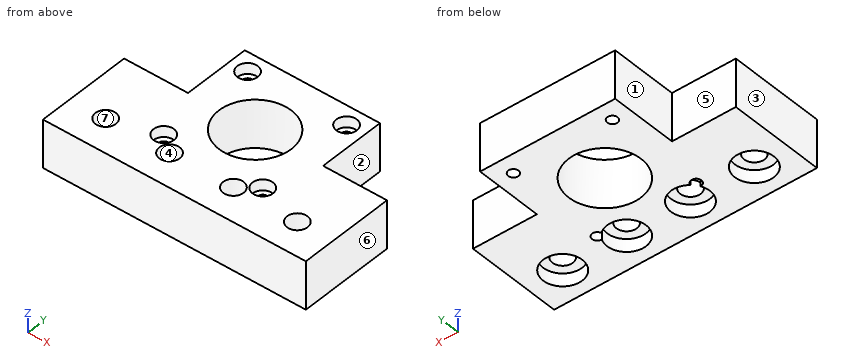
from build123d import *

# Parameters (mm, degrees)
SKETCH_R        = 11.3
SKETCH_R_2      = 1.6
SKETCH_R_3      = 3.2
PAD_DEPTH       = 15
SKETCH001_R     = 3.2
POCKET_DEPTH    = 3.4
SKETCH002_R     = 6.1
POCKET001_DEPTH = 4


with BuildPart() as part:
    # Sketch → Pad (new body)
    with BuildSketch(Plane.XY):
        Polygon((20, 30), (20, 51), (62.3, 51), (62.3, 30), (82.3, 30), (82.3, 0), (0, 0), (0, 30), align=None)
        with Locations((41.15, 29.85)):
            Circle(SKETCH_R, mode=Mode.SUBTRACT)
        with Locations((25.65, 45.35)):
            Circle(SKETCH_R_2, mode=Mode.SUBTRACT)
        with Locations((25.65, 14.35)):
            Circle(SKETCH_R_2, mode=Mode.SUBTRACT)
        with Locations((56.65, 45.35)):
            Circle(SKETCH_R_2, mode=Mode.SUBTRACT)
        with Locations((56.65, 14.35)):
            Circle(SKETCH_R_2, mode=Mode.SUBTRACT)
        with Locations((11.15, 10)):
            Circle(SKETCH_R_3, mode=Mode.SUBTRACT)
        with Locations((31.15, 10)):
            Circle(SKETCH_R_3, mode=Mode.SUBTRACT)
        with Locations((51.15, 10)):
            Circle(SKETCH_R_3, mode=Mode.SUBTRACT)
        with Locations((71.15, 10)):
            Circle(SKETCH_R_3, mode=Mode.SUBTRACT)
    extrude(amount=PAD_DEPTH)

    # Sketch001 (on Face19 of Pad) → Pocket (cut)
    with BuildSketch(Plane.XY.offset(15)):
        with Locations((25.65, 45.35)):
            Circle(SKETCH001_R)
        with Locations((56.65, 45.35)):
            Circle(SKETCH001_R)
        with Locations((56.65, 14.35)):
            Circle(SKETCH001_R)
        with Locations((25.65, 14.35)):
            Circle(SKETCH001_R)
    extrude(amount=-POCKET_DEPTH, mode=Mode.SUBTRACT)

    # Sketch002 (on Face4 of Pocket) → Pocket001 (cut)
    with BuildSketch(Plane(origin=(0, 0, 0), x_dir=(1, 0, 0), z_dir=(0, 0, -1))):
        with Locations((11.15, -10)):
            Circle(SKETCH002_R)
        with Locations((31.15, -10)):
            Circle(SKETCH002_R)
        with Locations((51.15, -10)):
            Circle(SKETCH002_R)
        with Locations((71.15, -10)):
            Circle(SKETCH002_R)
    extrude(amount=-POCKET001_DEPTH, mode=Mode.SUBTRACT)


solid = part.part
Read the model definition and answer for the solid it produces. Units are mm, in the model's axes. Face numbers are marked on the shaded views. A direction names the side the tool comes from. Round coordinates to 2 decimals unless told otherwise and drop trailing zeros. Loops run counter-clockwise (first coordinate to the right, second up) from the corner with the lowest first, then second, coordinate; pieces in that order, holes last.
Q1. Section A-A on x = 41.15 is taken. Write down the section's boundary in (y, z).
Q2. Which of the six approach directions +Z, -Z, +X, -X, +Y, -Y give full straight-line access (tool end or side, diameter ignored) to the marked faces 1, 2 and 3?
Q3. Section B-B on y = 45.35 is taken. Write down the section's boundary in (x, z).
Q4. Section D-D on y = 35 is taken. Write down the section's boundary in (x, z).
Q5. Section C-C on z = 7.75 is taken. Give the number of separate pieces and of enclosed holes in the cut face, and give its area (3 significant figures).
Q6. Determine the mould class of the marked faces 4, 5, 6 and 7 for opening direction Y: released by +Y, released by -Y, zero draft, split by the parting line, or undercut.
Q7. Each of these flat-tipped pins is pushed along its axis until it touches: pin 1 (10 mm diameter, centred on x = 11, y = 9, fed in from -Z); pin 2 (1.5 mm diameter, centred on y = 43.5, z = 9.5, fed in from +X); pin 3 (1.9 mm diameter, centred on x = 56, y = 14, fed in from +Z). Where does it stop, or does it pass through?
Q8. Consider probe 1 along X at (y, z) = (14.35, 9.25); probe 2 along X at (y, z) = (10, 2.6); probe 3 along Y at (x, z) = (25.65, 6.5). Determine where each line is inside the solid, lowest interval first.
Output:
1. outline: (0, 0) - (18.55, 0) - (18.55, 15) - (0, 15) - close; (41.15, 0) - (51, 0) - (51, 15) - (41.15, 15) - close
2. face 1: +Z, -Z, -X, +Y
2. face 2: +Z, -Z, +X, +Y
2. face 3: +Z, -Z, -X, +Y, -Y
3. outline: (20, 0) - (24.05, 0) - (24.05, 11.6) - (22.45, 11.6) - (22.45, 15) - (20, 15) - close; (27.25, 0) - (55.05, 0) - (55.05, 11.6) - (53.45, 11.6) - (53.45, 15) - (28.85, 15) - (28.85, 11.6) - (27.25, 11.6) - close; (58.25, 0) - (62.3, 0) - (62.3, 15) - (59.85, 15) - (59.85, 11.6) - (58.25, 11.6) - close
4. outline: (20, 0) - (31.09, 0) - (31.09, 15) - (20, 15) - close; (51.21, 0) - (62.3, 0) - (62.3, 15) - (51.21, 15) - close
5. separate pieces: 1
5. enclosed holes: 9
5. area: 2,800 mm2
6. face 4: undercut
6. face 5: released by +Y
6. face 6: zero draft
6. face 7: undercut
7. pin 1: stops at z = 4
7. pin 2: stops at x = 62.3
7. pin 3: stops at z = 11.6
8. probe 1: x = 0 to 24.05, 27.25 to 55.05, 58.25 to 82.3
8. probe 2: x = 0 to 5.05, 17.25 to 25.05, 37.25 to 45.05, 57.25 to 65.05, 77.25 to 82.3
8. probe 3: y = 0 to 12.75, 15.95 to 43.75, 46.95 to 51
